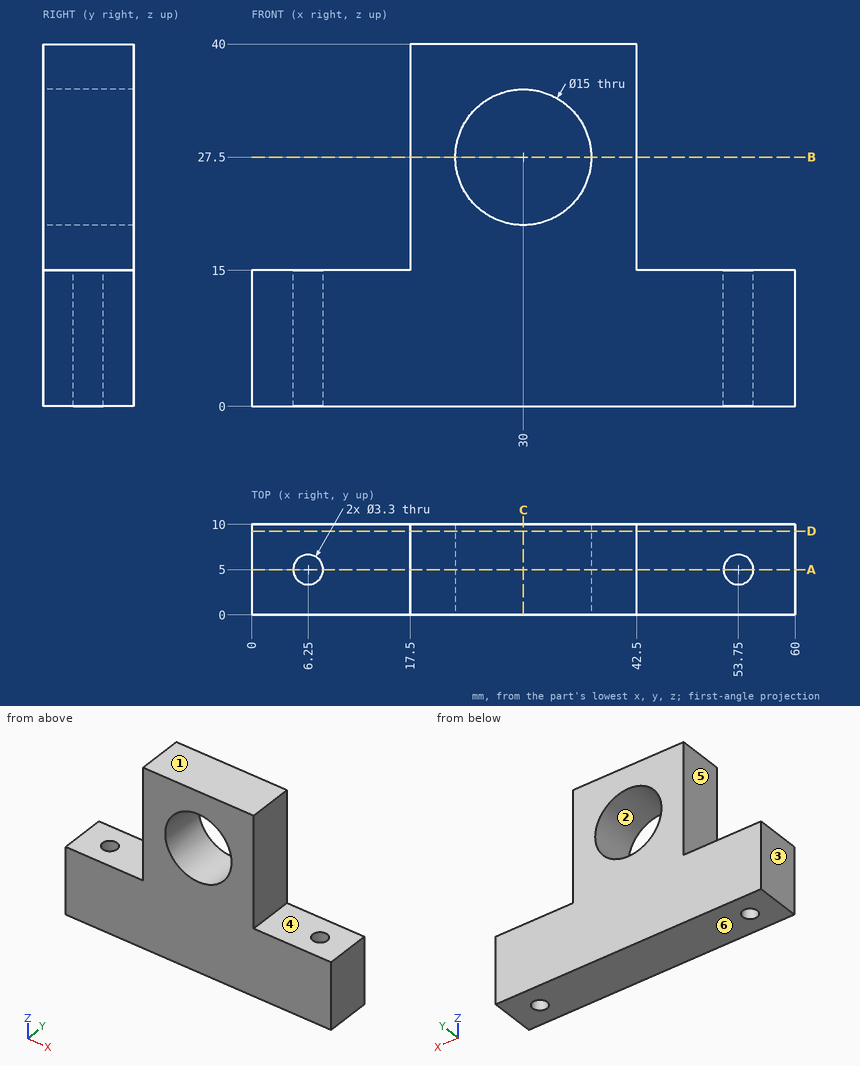
Geometry check sheet. Reference: drawing and pictorial views, mm from the part's lowest x, y, z. A direction names the side the tool comes from. Give positions to 0.01 mm unless a question says otherwise; leave off trailing zeros. Order: outer loops, then holes, each group sorted by start corner. A loop starts at its lowest first (then second) coordinate and runs counter-clockwise, first axis right, second up. Notation, with made-up numbers: M 22.5,42 L 58.5,42 A26 cw 58.5,68 Z; hole C -25,30 d1. An arc over 180 degrees is marked long. Answer in a Markdown table with one row per item. Add a question column.
Item 1: Section check A-A, the plane y = 5. Enter the section's corners in (x, z).
Item 2: Section check B-B, the plane z = 27.5. Enter the section's corners in (x, y), and give its area (3 significant figures).
Item 3: Mould release check, pull along X, two halves, no side actions. Record for the marked faces 1, 2 and 3: released by +X, released by -X, zero draft, split by the parting line, or undercut.
Item 4: Gauge pin test, flat ends, axial feed: pin 1 (3 mm diameter, centred on x = 6.25, y = 5, fed in from -Z); pin 2 (3 mm diameter, centred on y = 7.5, z = 31.5, fed in from -X); pin 3 (3 mm diameter, centred on x = 53, y = 6, fed in from +Z). Record the tip position at first contact, or that the pin passes through.
Item 5: Scan lines: probe 1 along X at (y, z) = (4.25, 27.5); probe 2 along Y at (x, z) = (53.75, 7.25); probe 3 along Z at (x, y) = (15.5, 1.5). Record each from-to range of solid material in increasing order. Write a range as from..to.
Item 6: Section check C-C, the plane x = 30. Enter the section's corners in (y, z).
Item 7: Section check D-D, the plane y = 9.25. Enter the section's corners in (x, z).
Item 8: Tool access check on the marked faces 4, 5 and 6. Record the directions out of +Z, -Z, +X, -X, +Y, -Y that give a thin tool (end or side, any length) a straight path to the whole face; none if there is none.
Filled sheet:
| question | item | result |
|---|---|---|
| 1 | outline | M 0,0 L 4.6,0 L 4.6,15 L 0,15 Z; M 7.9,0 L 52.1,0 L 52.1,15 L 42.5,15 L 42.5,40 L 17.5,40 L 17.5,15 L 7.9,15 Z; M 55.4,0 L 60,0 L 60,15 L 55.4,15 Z; hole C 30,27.5 d15 |
| 2 | outline | M 17.5,0 L 22.5,0 L 22.5,10 L 17.5,10 Z; M 37.5,0 L 42.5,0 L 42.5,10 L 37.5,10 Z |
| 2 | area | 100 mm^2 |
| 3 | face 1 | zero draft |
| 3 | face 2 | undercut |
| 3 | face 3 | released by -X |
| 4 | pin 1 | passes through |
| 4 | pin 2 | stops at x = 17.5 |
| 4 | pin 3 | stops at z = 15 |
| 5 | probe 1 | x = 17.5..22.5, 37.5..42.5 |
| 5 | probe 2 | y = 0..3.35, 6.65..10 |
| 5 | probe 3 | z = 0..15 |
| 6 | outline | M 0,0 L 10,0 L 10,20 L 0,20 Z; M 0,35 L 10,35 L 10,40 L 0,40 Z |
| 7 | outline | M 0,0 L 60,0 L 60,15 L 42.5,15 L 42.5,40 L 17.5,40 L 17.5,15 L 0,15 Z; hole C 30,27.5 d15 |
| 8 | face 4 | +Z, +X, +Y, -Y |
| 8 | face 5 | +Z, -X, +Y, -Y |
| 8 | face 6 | -Z, +X, -X, +Y, -Y |
